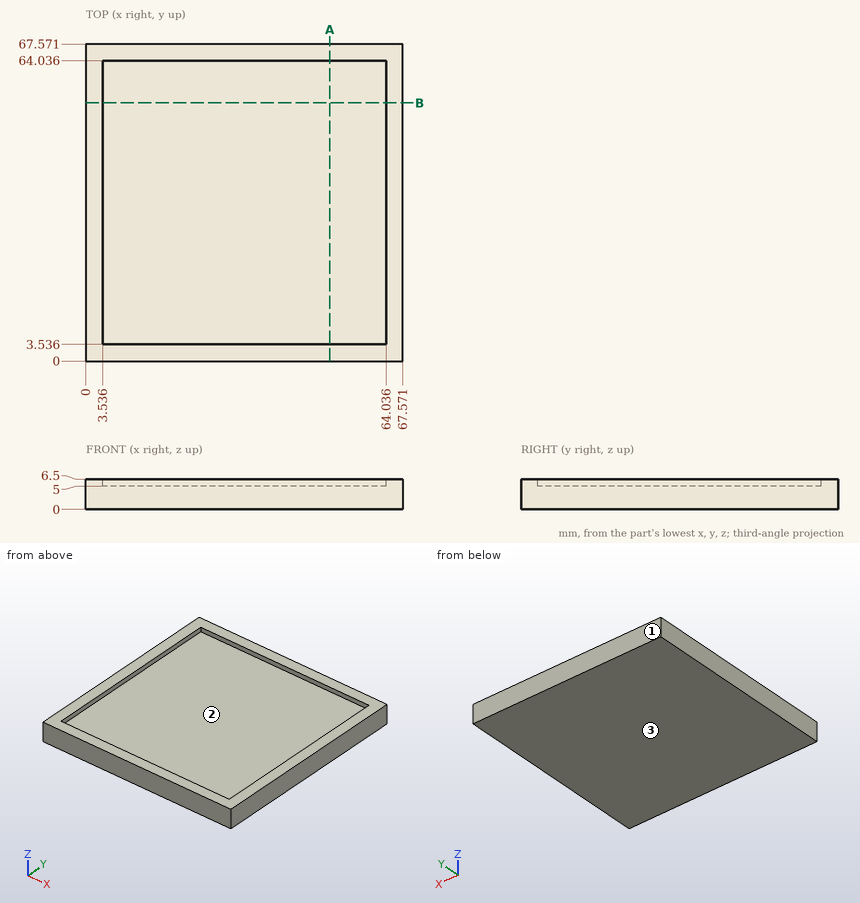
Here's the drawing with two shaded views (mm, measured from the low corner). I have some questions. Give positions to 0.01 mm unless a question says otherwise; leave off trailing zeros. Order: outer loops, then holes, each group sorted by start corner. A loop starts at its lowest first (then second) coordinate and runs counter-clockwise, first axis right, second up.
Q1. I'm going to push a flat-ended pin straight in: P1, Ø18, axis at x = 20, y = 37.5, coming from the +Z side. Where does the tip first touch, or does it pass through?
Q2. Suppose I cut it at A-A, the plane x = 52. Write out the boundary of the cut face in (y, z) (1 decimal).
Q3. If I drill on line 1 along Y through (x, z) = (34.5, 5.5) (1 decimal); line 2 along Z through (x, y) = (38, 40), over which ranges is the centre line in solid material (lowest first)?
Q4. We'd pull the mould along Y, two halves only. Please class the marked faces 1, 2 and 3: +Y half, -Y half, draft (parallel to the pull), parting line (faces both ways), or undercut.
Solution:
1. P1: stops at z = 5
2. outline: (0, 0) - (67.6, 0) - (67.6, 6.5) - (64, 6.5) - (64, 5) - (3.5, 5) - (3.5, 6.5) - (0, 6.5) - close
3. line 1: y = 0 to 3.5, 64 to 67.6
3. line 2: z = 0 to 5
4. face 1: +Y half
4. face 2: undercut
4. face 3: draft
